Autodesk Inventor part; units mm, degrees
ref_plane "Work Plane1" through (0, 0, 2.5) normal (0, 0, 1) x (1, 0, 0)
ref_plane "YZ Plane" through (0, 0, 0) normal (1, 0, 0) x (0, 1, 0)
ref_plane "XZ Plane" through (0, 0, 0) normal (0, 1, 0) x (-1, 0, 0)
sketch "Sketch1" plane through (0, 0, 0) normal (0, 0, 1) x (1, 0, 0)
  circle A0 centre (0, 4) radius 2
  circle A1 centre (-4, 0) radius 2
  circle A2 centre (0, -4) radius 2
  circle A3 centre (4, 0) radius 2
  line L0 (8, 11.7321) -> (15.5744, 40)
  line L1 (7, 8) -> (40.1288, 8) construction
  line L2 (-8, 11.7321) -> (-15.5744, 40)
  line L3 (8, 0) -> (8, 11.7321)
  line L4 (-8, 0) -> (-8, 11.7321)
  arc A4 (-8, 0) -> (8, 0) centre (0, 0) ccw
  line L5 (0, 43) -> (16.3782, 43)
  line L6 (16.3782, 43) -> (15.5744, 40)
  line L7 (-15.5744, 40) -> (-16.3782, 43)
  line L8 (-16.3782, 43) -> (0, 43)
  dimension "d2" = 4
  dimension "d5" = 360
extrude "Extrusion1" add sketch "Sketch1" along normal blind 5
sketch "Sketch2" plane through (0, 0, 0) normal (0, 0, -1) x (-1, 0, 0)
  circle A0 centre (0, 0) radius 6.625
  dimension "d18" = 13.25
extrude "Extrusion2" cut sketch "Sketch2" against normal blind 2
sketch "Sketch4" plane through (0, 0, 0) normal (0, 0, -1) x (-1, 0, 0)
  line L0 (-8, 11.7321) -> (-16.3782, 43)
  line L1 (-16.3782, 43) -> (16.3782, 43)
  line L2 (-16.3782, 43) -> (16.3782, 43)
  line L3 (0, 39.136) -> (15.3429, 39.136)
  line L4 (16.3782, 43) -> (8, 11.7321)
  line L5 (15.3429, 39.136) -> (16.3782, 43)
  line L6 (0, 39.136) -> (-15.3429, 39.136)
  line L7 (-15.3429, 39.136) -> (-16.3782, 43)
  point P0 (0, 0)
extrude "Extrusion4" add sketch "Sketch4" along normal blind 73.5
sketch "Sketch5" plane through (-16.3782, 43, 5) normal (0, 1, 0) x (1, 0, 0)
  line L0 (0, 78.5) -> (32.7564, 78.5)
  line L1 (32.7564, 0) -> (0, 0)
  line L2 (0, 78.5) -> (32.7564, 78.5)
  line L3 (32.7564, 78.5) -> (32.7564, 0)
  line L4 (32.7564, 0) -> (0, 0)
  line L5 (0, 0) -> (0, 78.5)
  point P0 (16.3782, 5)
extrude "Extrusion5" add sketch "Sketch5" along normal blind 30
sketch "Sketch6" plane through (16.3782, 43, -73.5) normal (1, 0, 0) x (0, 0, -1)
  line L0 (-78.5, 30) -> (0, 30)
  line L1 (-39.25, 30) -> (-26.55, 30)
  line L2 (-39.25, 30) -> (-51.95, 30)
  line L3 (-51.95, 30) -> (-54.95, 30)
  line L4 (-26.55, 30) -> (-23.55, 30)
  line L5 (0, -3.864) -> (0, 0)
  line L6 (-23.55, 30) -> (0, 0)
  line L7 (0, 0) -> (0, 30)
  line L8 (0, 0) -> (0, 30)
  line L9 (0, 30) -> (-23.55, 30)
  line L10 (-54.95, 30) -> (-78.5, 30)
  line L11 (-78.5, 0) -> (-78.5, 30)
  line L12 (-78.5, 30) -> (-78.5, 0)
  line L13 (-78.5, 0) -> (-54.95, 30)
  point P0 (-73.5, -43)
  dimension "d30" = 12.7
  dimension "d31" = 12.7
  dimension "d32" = 3
  dimension "d33" = 3
extrude "Extrusion6" cut sketch "Sketch6" against normal up to surface (32.7564 mm away)
sketch "Sketch7" plane through (-16.3782, 73, 5) normal (0, 1, 0) x (1, 0, 0)
  line L0 (0, 78.5) -> (0, 0)
  line L1 (0, 23.55) -> (32.7564, 23.55)
  line L2 (16.3782, 52.25) -> (3.3782, 52.25)
  line L3 (3.3782, 52.25) -> (3.3782, 26.25)
  line L4 (3.3782, 26.25) -> (29.3782, 26.25)
  line L5 (29.3782, 26.25) -> (29.3782, 52.25)
  line L6 (29.3782, 52.25) -> (16.3782, 52.25)
  point P0 (16.3782, 5)
  dimension "d37" = 13
  dimension "d38" = 26
  dimension "d39" = 26
extrude "Extrusion7" cut sketch "Sketch7" against normal blind 25.4
ref_plane "Work Plane1" through (0, 0, 2.5) normal (0, 0, 1) x (1, 0, 0)
sketch "Sketch8" plane through (0, 0, 2.5) normal (0, 0, 1) x (1, 0, 0)
  line L0 (16.3782, 43) -> (-16.3782, 43)
  circle A0 centre (0, 53) radius 2
  point P0 (0, 0)
  dimension "d43" = 4
extrude "Extrusion8" cut sketch "Sketch8" against normal through all
sketch "Sketch9" plane through (16.3782, 43, 5) normal (1, 0, 0) x (0, 0, -1)
  line L0 (26.25, 30) -> (52.25, 30)
  circle A0 centre (39.25, 20) radius 2
  point P0 (5, -43)
  dimension "d47" = 4
extrude "Extrusion9" cut sketch "Sketch9" against normal up to surface (32.7564 mm away)
sketch "Sketch10" plane through (8, 0, 0) normal (1, 0, 0) x (0, 0, -1)
  line L0 (0, 39.136) -> (73.5, 39.136)
  line L1 (-5, 0) -> (-5, -8)
  line L2 (0, 39.136) -> (-5, 39.136)
  line L3 (-5, 39.136) -> (-5, -8)
  line L4 (-5, -8) -> (0, -8)
  line L5 (0, -8) -> (0, 39.136)
  point P0 (0, 0)
extrude "Extrusion10" cut sketch "Sketch10" along normal blind 10 and the other way blind 25
properties part number "Second_Tilt_Motor_Mount"
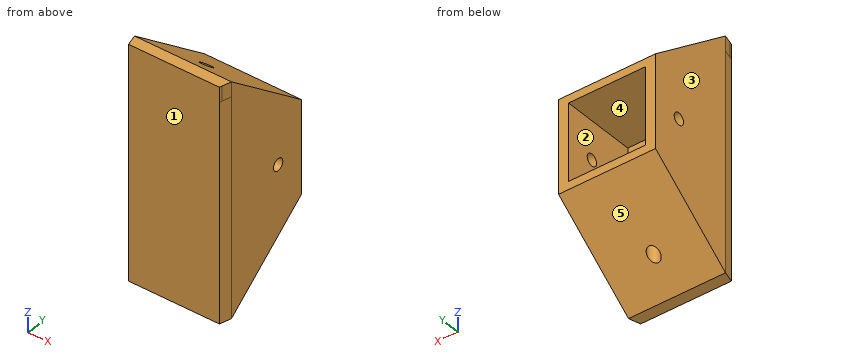
For this review, take the finished solid that the model builds, in its own axes (mm). Face numbers are marked on the shaded views. A direction names the side the tool comes from. Give positions to 0.01 mm unless a question says otherwise; leave off trailing zeros. Loops run counter-clockwise (first coordinate to the right, second up) from the corner with the lowest first, then second, coordinate; pieces in that order, holes last. Notation, with made-up numbers: M 37.5,81 L 54.5,81 A9 ccw 54.5,98 Z; hole C -14,22.25 d1. An arc over 180 degrees is marked long. One line per item, written item: value. Start each with the question number.
Q1. Draft analysis for pull direction Z (two halves, no side actions). For the marked faces 3, 4 and 5, state which applies: released by +Z, released by -Z, zero draft, split by the parting line, or undercut.
Q2. Machinability: for the marked faces 1 and 2, which of the approach directions +Z, -Z, +X, -X, +Y, -Y give a long, thin tool a straight path to every point of the face, cutting with its end or side? Answer none if there is none.
Q3. Add section D-D (y = 58). Give the boundary of the cut face in (x, z) (3 decimals).
Q4. Add section A-A (y = 63). Give the boundary of the cut face in (x, z), and give its area (3 significant figures).
Q5. Add section C-C (x = 7.5). Give the boundary of the cut face in (y, z).
Q6. Clearance check with flat-ended pins moving along their axes: pin 1 Ø8 at (x, z) = (6, -34.5) entering from +Y; pin 2 Ø10 at (x, y) = (-1, 63) entering from +Z (3 decimals); pin 3 Ø7.5 at (x, y) = (5.5, 62.5) entering from +Z; pin 4 Ø2.5 at (y, z) = (63, -34.25) entering from -X. State where each tip first meets the part, or that it passes through.
Q7. Add section B-B (x = 0). Give the boundary of the cut face in (y, z).
Q8. For L1, parallel to X at y = 71, z = -39.5; L2, parallel to X at y = 53, z = -16; L3, parallel to Y at x = -14, z = -34.25, list the stretches that pass through material, from the lowest coordinate up.
Reply:
1. face 3: zero draft
1. face 4: undercut
1. face 5: released by -Z
2. face 1: +Z, -Z, +X, -X, -Y
2. face 2: +Y
3. outline: M -16.378,-61.725 L 16.378,-61.725 L 16.378,-6.775 L -16.378,-6.775 Z; hole M -13,-47.25 L 13,-47.25 L 13,-21.25 L -13,-21.25 Z
4. outline: M -16.38,-57.8 L 16.38,-57.8 L 16.38,-36.25 L 13,-36.25 L 13,-47.25 L -13,-47.25 L -13,-36.25 L -16.38,-36.25 Z; M -16.38,-32.25 L -13,-32.25 L -13,-21.25 L 13,-21.25 L 13,-32.25 L 16.38,-32.25 L 16.38,-10.7 L -16.38,-10.7 Z
4. area: 840 mm²
5. outline: M 39.14,-73.5 L 43,-73.5 L 73,-49.95 L 73,-47.25 L 47.6,-47.25 L 47.6,-21.25 L 73,-21.25 L 73,-18.55 L 43,5 L 39.14,5 Z
6. pin 1: y = 47.6
6. pin 2: z = -6.775
6. pin 3: z = -7.36
6. pin 4: through
7. outline: M 39.14,-73.5 L 43,-73.5 L 51,-67.22 L 51,-47.25 L 47.6,-47.25 L 47.6,-21.25 L 51,-21.25 L 51,-1.28 L 43,5 L 39.14,5 Z; M 55,-64.08 L 73,-49.95 L 73,-47.25 L 55,-47.25 Z; M 55,-21.25 L 73,-21.25 L 73,-18.55 L 55,-4.42 Z
8. L1: -16.38 to -13, 13 to 16.38
8. L2: -16.38 to -2, 2 to 16.38
8. L3: 39.14 to 61, 65 to 73
